Could you check a few things on this model? Use its own coordinates, in mm. Face numbers are marked on the shaded views. A direction names the side the tool comes from. Give positions to 0.01 mm unless a question says otherwise; leave off trailing zeros. Write each loop counter-clockwise with the first axis right and the second up, starting at its lowest first coordinate (ties: lowest second). Pieces come first, ordered by that corner, then holes. Notation, with made-up numbers: M 87.5,-22.5 L 94.5,-22.5 A24 ccw 94.5,-5.5 Z; hole C 0,3 d3. An arc over 180 degrees is marked long. Use one line per item in the form item = value.
from build123d import *

# Parameters (mm, degrees)
F2_R     = 9.9
F3_DEPTH = 27
F4_R     = 6.5
F5_DEPTH = 4.5
F6_R     = 3.25
F7_DEPTH = 22.501


with BuildPart() as f3:
    # F2 (on Top) → F3 (new body)
    with BuildSketch(Plane.XY):
        Circle(F2_R)
    extrude(amount=F3_DEPTH)

    # F4 (on face) → F5 (cut)
    with BuildSketch(Plane.XY.offset(27)):
        Circle(F4_R)
    extrude(amount=-F5_DEPTH, mode=Mode.SUBTRACT)

    # F6 (on face) → F7 (cut, through all)
    with BuildSketch(Plane.XY.offset(22.5)):
        Circle(F6_R)
    extrude(amount=-F7_DEPTH, mode=Mode.SUBTRACT)

    # F8: F3 across plane


with BuildPart() as f3_1:
    add(f3.part)
    add(f3.part.mirror(Plane.XY))


solid = f3_1.part
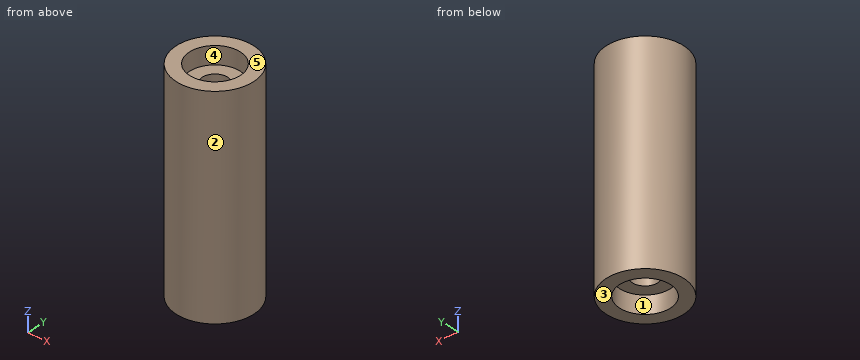
1) For pin 1 Ø1 at (y, z) = (-5.5, -14) entering from +X; pin 2 Ø4 at (x, y) = (-2, -1) entering from -Z; pin 3 Ø3 at (x, z) = (-7, 12) entering from -Y; pin 4 Ø5 at (x, y) = (0, 0) entering from +Z, each with a flat end and sliding along its axis, tell me the tip position at first contact or that it passes through.
Checked values:
pin_1 = 8.54
pin_2 = -22.5
pin_3 = -8.23
pin_4 = through
2) I want a section at D-D, the plane x = -4.5. Please give me the cut outline in (y, z).
Checked values:
outline = M -8.82,-27 L -4.69,-27 L -4.69,-22.5 L 4.69,-22.5 L 4.69,-27 L 8.82,-27 L 8.82,27 L 4.69,27 L 4.69,22.5 L -4.69,22.5 L -4.69,27 L -8.82,27 Z
3) I want a section at A-A, the plane x = 0. Please give me the cut outline in (y, z).
Checked values:
outline = M -9.9,-27 L -6.5,-27 L -6.5,-22.5 L -3.25,-22.5 L -3.25,22.5 L -6.5,22.5 L -6.5,27 L -9.9,27 Z; M 3.25,-22.5 L 6.5,-22.5 L 6.5,-27 L 9.9,-27 L 9.9,27 L 6.5,27 L 6.5,22.5 L 3.25,22.5 Z
4) I want a section at C-C, the plane z = 3.5. Please give me the cut outline in (x, y), plus the area to 3 significant figures.
Checked values:
outline = C 0,0 d19.8; hole C 0,0 d6.5
area = 275 mm2
5) For the marked faces 4 and 5, which set-ups out of +Z, -Z, +X, -X, +Y, -Y let a thin tool reach every point of the face, with its end or its side?
Checked values:
face_4 = +Z
face_5 = +Z, +X, -X, +Y, -Y
6) If I drill on L1, parallel to Y at x = 0, z = -23.4; L2, parallel to Y at x = 0, z = -6; L3, parallel to X at y = 2.25, z = 23, over which ranges is the centre line in solid material (lowest first)?
Checked values:
L1 = -9.9 to -6.5, 6.5 to 9.9
L2 = -9.9 to -3.25, 3.25 to 9.9
L3 = -9.64 to -6.1, 6.1 to 9.64
7) Thinking about a two-plate mould opening in X: for the marked faces 1, 2 and 3, which applies, released by +X, released by -X, zero draft, split by the parting line, or undercut?
Checked values:
face_1 = undercut
face_2 = split by the parting line
face_3 = zero draft
